Autodesk Inventor part; units mm, degrees
ref_plane "YZ Plane" through (0, 0, 0) normal (1, 0, 0) x (0, 1, 0)
ref_plane "XZ Plane" through (0, 0, 0) normal (0, 1, 0) x (-1, 0, 0)
ref_plane "XY Plane" through (0, 0, 0) normal (0, 0, 1) x (1, 0, 0)
sketch "Esquisse1" plane through (0, 0, 0) normal (0, 0, 1) x (1, 0, 0)
  line L0 (0, 0) -> (-27.546, -25.0426) construction
  line L1 (0, 0) -> (23.0277, -27.4577) construction
  circle A0 centre (-18.0975, -16.4528) radius 1.25
  circle A1 centre (15.7127, -18.7355) radius 1.25
  arc A2 (-16.6894, -17.8731) -> (14.1299, -19.9581) centre (0, 0) ccw
  arc A3 (-16.6894, -17.8731) -> (-19.3824, -14.9201) centre (-18.0975, -16.4528) ccw
  arc A4 (17.0433, -17.2424) -> (14.1299, -19.9581) centre (15.7127, -18.7355) ccw
  line L2 (0, 0) -> (-29.5508, 10.7556) construction
  line L3 (-17.8311, 0) -> (17.1748, 0) construction
  line L4 (0, 2.0526) -> (0, -2.2236) construction
  line L5 (-28.8657, 0) -> (-36, 0)
  line L6 (28.8657, 0) -> (36, 0)
  line L7 (36, 0) -> (36, -2)
  line L8 (36, -2) -> (25.923, -2)
  line L9 (-36, 0) -> (-36, -2)
  line L10 (-36, -2) -> (-25.923, -2)
  arc A5 (-25.923, -2) -> (25.923, -2) centre (0, 0) ccw
  circle A6 centre (0, 0) radius 22.5 construction
  arc A7 (-16.6894, -17.8731) -> (14.1299, -19.9581) centre (0, 0) ccw
  arc A8 (-16.6894, -17.8731) -> (14.1299, -19.9581) centre (0, 0) ccw
  circle A9 centre (-25.3169, 1.1605) radius 1.25
  circle A10 centre (25.3169, 1.1605) radius 1.25
  line L11 (24.0891, 2.7784) -> (24.0891, 12.8348)
  line L12 (25.8363, 12.8348) -> (24.0891, 12.8348)
  line L13 (-25.923, 6.143) -> (-25.923, 12.7847)
  line L14 (-24.2942, 2.9148) -> (-24.2942, 12.7847)
  line L15 (-24.2942, 12.7847) -> (-25.923, 12.7847)
  arc A11 (-24.4506, -0.676) -> (-19.3824, -14.9201) centre (0, 0) ccw
  arc A12 (-24.4506, -0.676) -> (-19.3824, -14.9201) centre (0, 0) ccw
  arc A13 (-24.4506, -0.676) -> (-24.2942, 2.9148) centre (-25.3169, 1.1605) ccw
  arc A14 (17.0433, -17.2424) -> (24.2376, -0.5599) centre (0, 0) ccw
  arc A15 (17.0433, -17.2424) -> (24.2376, -0.5599) centre (0, 0) ccw
  arc A16 (17.0433, -17.2424) -> (24.2376, -0.5599) centre (0, 0) ccw
  arc A17 (24.0891, 2.7784) -> (24.2376, -0.5599) centre (25.3169, 1.1605) ccw
  line L16 (-28.8657, 0) -> (-25.923, 6.143)
  line L17 (28.8657, 0) -> (25.923, 6.143)
  line L18 (25.8363, 3.0919) -> (25.8363, 3.124)
  line L19 (25.8363, 6.3239) -> (25.8363, 12.8348)
  line L20 (25.8363, 6.3239) -> (28.8657, 0)
  point P0 (-26.3114, 9.5766)
  dimension "d35" = 2.5
  dimension "d36" = 2.5
  dimension "d37" = 4
  dimension "d38" = 4
  dimension "d39" = 20
  dimension "d44" = 2
  dimension "d45" = 2
  dimension "d52" = 45
  dimension "d65" = 2.5
ref_plane "Plan de construction1" through (-42, 0, 0) normal (0, 1, 0) x (1, 0, 0)
ref_plane "Plan de construction2" through (-36, 0, 0) normal (0, 1, 0) x (1, 0, 0)
sketch "Esquisse3" plane through (-36, 0, 0) normal (0, 1, 0) x (1, 0, 0)
  line L0 (0, 0) -> (10, 0)
  line L1 (0, 0) -> (0, -8)
  line L2 (10, -8) -> (0, -8)
  line L3 (10, 0) -> (10, -8)
  circle A0 centre (4, -4) radius 2.15
  line L4 (62, 0) -> (72, 0)
  line L5 (62, 0) -> (62, -8)
  line L6 (72, -8) -> (62, -8)
  line L7 (72, 0) -> (72, -8)
  circle A1 centre (68, -4) radius 2.15
  point P0 (36, 0)
  dimension "d48" = 4.3
  dimension "d73" = 4
  dimension "d74" = 4.3
  dimension "d75" = 4
extrude "Extrusion14" add sketch "Esquisse1" along normal blind 8
extrude "Extrusion15" cut sketch "Esquisse3" against normal blind 8 contours A0 | A1
sketch "Esquisse4" plane through (0, 0, 8) normal (0, 0, 1) x (1, 0, 0)
  circle A0 centre (25.3169, 1.1605) radius 1.25
  circle A1 centre (-25.3169, 1.1605) radius 1.25
  circle A2 centre (15.7127, -18.7355) radius 1.25
  circle A3 centre (-18.0975, -16.4528) radius 1.25
  arc A4 (-16.6894, -17.8731) -> (-19.3824, -14.9201) centre (-18.0975, -16.4528) ccw
  arc A5 (-24.4506, -0.676) -> (-19.3824, -14.9201) centre (0, 0) ccw
  arc A6 (-24.4506, -0.676) -> (-24.2942, 2.9148) centre (-25.3169, 1.1605) ccw
  line L0 (-24.2942, 2.9148) -> (-24.2942, 12.7847)
  line L1 (-24.2942, 12.7847) -> (-25.923, 12.7847)
  line L2 (-25.923, 12.7847) -> (-25.923, 6.143)
  line L3 (-25.923, 6.143) -> (-28.8657, 0)
  line L4 (-28.8657, 0) -> (-36, 0)
  line L5 (-36, 0) -> (-36, -2)
  line L6 (-36, -2) -> (-25.923, -2)
  arc A7 (-25.923, -2) -> (25.923, -2) centre (0, 0) ccw
  line L7 (25.923, -2) -> (36, -2)
  line L8 (36, -2) -> (36, 0)
  line L9 (36, 0) -> (28.8657, 0)
  line L10 (28.8657, 0) -> (25.8363, 6.3239)
  line L11 (25.8363, 6.3239) -> (25.8363, 12.8348)
  line L12 (25.8363, 12.8348) -> (24.0891, 12.8348)
  line L13 (24.0891, 12.8348) -> (24.0891, 2.7784)
  arc A8 (24.0891, 2.7784) -> (24.2376, -0.5599) centre (25.3169, 1.1605) ccw
  arc A9 (17.0433, -17.2424) -> (24.2376, -0.5599) centre (0, 0) ccw
  arc A10 (17.0433, -17.2424) -> (14.1299, -19.9581) centre (15.7127, -18.7355) ccw
  arc A11 (-16.6894, -17.8731) -> (14.1299, -19.9581) centre (0, 0) ccw
  dimension "d78" = 2.5
properties part number "anneau"
The model under review builds one solid part; all positions refer to its coordinate system, in mm. A direction names the side the tool comes from. Round coordinates to 2 decimals unless told otherwise and drop trailing zeros. Loops run counter-clockwise (first coordinate to the right, second up) from the corner with the lowest first, then second, coordinate; pieces in that order, holes last. Notation, with made-up numbers: M -14,61.25 L -2,61.25 A31 ccw -2,100.25 Z; hole C -36.75,72 d9. An arc over 180 degrees is marked long. Answer as a JSON object with one key per item and string values.
(1) Take a section at A-A on x = -32. Give the boundary of the cut face in (y, z).
Resolved:
{"outline": "M -2,0 L 0,0 L 0,1.85 L -2,1.85 Z; M -2,6.15 L 0,6.15 L 0,8 L -2,8 Z"}
(2) Take a section at B-B on y = 8. Give the boundary of the cut face in (x, z), and give its area (3 significant figures).
Resolved:
{"outline": "M -25.92,0 L -24.29,0 L -24.29,8 L -25.92,8 Z; M 24.09,0 L 25.84,0 L 25.84,8 L 24.09,8 Z", "area": "27.0 mm²"}
(3) Take a section at C-C on z = 4. Count the separate pieces of the cut face and the enclosed holes in it, and give its area (3 significant figures).
Resolved:
{"separate pieces": "3", "enclosed holes": "4", "area": "208 mm²"}
(4) Draft analysis for pull direction X (two halves, no side actions). For faces 5 (the flat face through (-36, -1, 4)), 6 (the flat face through (0, -25, 8)), 7 (the cylindrical face through (-16.65, -15.07, 3.94)), state which applies: released by +X, released by -X, zero draft, split by the parting line, or undercut.
Resolved:
{"face 5": "released by -X", "face 6": "zero draft", "face 7": "undercut"}
(5) Take a section at D-D on z = 7. Give the boundary of the cut face in (x, y).
Resolved:
{"outline": "M -36,-2 L -25.92,-2 A26 ccw 25.92,-2 L 36,-2 L 36,0 L 28.87,0 L 25.92,6.14 L 25.84,6.32 L 25.84,12.83 L 24.09,12.83 L 24.09,2.78 A2.03 ccw 24.24,-0.56 A24.24 cw 17.04,-17.24 A2 ccw 14.13,-19.96 A24.45 cw -16.69,-17.87 A2 ccw -19.38,-14.92 A24.46 cw -24.45,-0.68 A2.03 ccw -24.29,2.91 L -24.29,12.78 L -25.92,12.78 L -25.92,6.14 L -28.87,0 L -36,0 Z; hole C -25.32,1.16 d2.5; hole C -18.1,-16.45 d2.5; hole C 15.71,-18.74 d2.5; hole C 25.32,1.16 d2.5"}
(6) Tool access review of faces 1 (the flat face through (-30, -2, 2)), 2 (the cylindrical face through (22.313, -9.481, 3.944)), 3 (the flat face through (30, -2, 2)), 4 (the flat face through (24.089, 8, 4)): name each direction out of +Z, -Z, +X, -X, +Y, -Y from which nothing blocks a thin tool from reaching the whole face with its end or side.
Resolved:
{"face 1": "+Z, -Z, -X, -Y", "face 2": "+Z, -Z", "face 3": "+Z, -Z, +X, -Y", "face 4": "+Z, -Z, +Y"}
(7) To check wall thickness, follow line 1 along X through (y, z) = (-0.45, 4); line 2 along X through (y, z) = (-1.5, 4.25); line 3 along X through (y, z) = (-4, 6). State the ranges of each line that lie inside material, in increasing order.
Resolved:
{"line 1": "-36 to -34.15, -29.85 to -24.08, 24.08 to 29.85, 34.15 to 36", "line 2": "-36 to -34.14, -29.86 to -24.41, 24.2 to 29.86, 34.14 to 36", "line 3": "-25.69 to -24.13, 23.91 to 25.69"}
(8) Clearance check with flat-ended pins moving along their axes: P1, Ø3.5, axis at x = -31, z = 3.5, coming from the +Y side; P2, Ø2, axis at y = -20.5, z = 5, coming from the -X side; P3, Ø1, axis at y = -12.5, z = 4.5, coming from the -X side. State where each tip first meets the part, or that it passes through.
Resolved:
{"P1": "y = 0", "P2": "x = -17.2", "P3": "x = -23.07"}
